Can you work these out from the model? Positions are in its coordinate system, mm. A direction names the side the tool comes from. Round coordinates to 2 decimals unless told otherwise and drop trailing zeros. Write each loop counter-clockwise with the first axis right and the second up, starting at its lowest first coordinate (ties: lowest second). Pieces come first, ordered by that corner, then holes. Notation, with made-up numbers: M 44,81.5 L 79,81.5 A19 cw 79,87.5 Z; hole C 17.5,-23.5 d2. An arc over 180 degrees is marked long. Answer in a Markdown table with one row per item. Add a question column.
(1) For faces 5 (the face through (21.15, 0, -18)), 6 (the face through (-2.38, 10.74, 1.01)), which set-ups out of +Z, -Z, +X, -X, +Y, -Y let a thin tool reach every point of the face, with its end or its side?
(2) Suppose I cut it at D-D, the plane x = -7.5. Write out the boundary of the cut face in (y, z).
(3) Suppose I cut it at A-A, the plane x = 0. Write out the boundary of the cut face in (y, z), then the cut area to 3 significant figures.
(4) If I drill on probe 1 along X at (y, z) = (-15.5, -24.5); probe 2 along Y at (x, z) = (-15, -17), over which ranges is the centre line in solid material (lowest first)?
(5) I'm going to push a flat-ended pin straight in: pin 1 (3 mm diameter, centred on x = 15.5, y = 15.5, fed in from +Z). Where does the tip first touch, or does it pass through?
(6) If we mould it in two halves opening along X, with no side actions, what happens to faces 1 (the face through (0, 0, 24)), 2 (the face through (14.579, -16.345, -18.487)), 3 (the face through (18.42, -18.35, -18.49)), 4 (the face through (-0.54, 2.44, 13.15))? For each: released by +X, released by -X, zero draft, split by the parting line, or undercut.
(7) Suppose I cut it at C-C, the plane z = 1. Write out the boundary of the cut face in (x, y), then the cut area to 3 significant figures.
from build123d import *

# Parameters (mm, degrees)
BOX002_W                    = 100
BOX002_H                    = 100
BOX002_DEPTH                = 37.5
COMPOUND002_PLACEMENT_ANGLE = 135
BOX003_W                    = 100
BOX003_H                    = 100
BOX003_DEPTH                = 37.5
COMPOUND003_PLACEMENT_ANGLE = 225
BOX004_W                    = 100
BOX004_H                    = 100
BOX004_DEPTH                = 37.5
COMPOUND004_PLACEMENT_ANGLE = 315
BOX001_W                    = 100
BOX001_H                    = 100
BOX001_DEPTH                = 37.5
COMPOUND001_PLACEMENT_ANGLE = 45
CYLINDER002_R               = 1.25
CYLINDER002_DEPTH           = 37.5
CYLINDER003_R               = 1.25
CYLINDER003_DEPTH           = 37.5
CYLINDER004_R               = 1.25
CYLINDER004_DEPTH           = 37.5
CYLINDER005_R               = 1.25
CYLINDER005_DEPTH           = 37.5
BOX_W                       = 42.3
BOX_H                       = 42.3
BOX_DEPTH                   = 37.5
CYLINDER_R                  = 11
CYLINDER_DEPTH              = 2
CYLINDER001_R               = 2.5
CYLINDER001_DEPTH           = 24
CUT001_PLACEMENT_ANGLE      = 180


with BuildPart() as compound002:
    # Box002 → Box002 (new body)
    with BuildSketch(Plane(origin=(26, -50, 0), x_dir=(1, 0, 0), z_dir=(0, 0, 1))):
        with Locations((50, 50)):
            Rectangle(BOX002_W, BOX002_H)
    extrude(amount=BOX002_DEPTH)


with BuildPart() as compound002_1:
    # Compound002 placement: moved
    add(compound002.part.rotate(Axis((0, 0, 0), (0, 0, 1)), COMPOUND002_PLACEMENT_ANGLE))


with BuildPart() as compound003:
    # Box003 → Box003 (new body)
    with BuildSketch(Plane(origin=(26, -50, 0), x_dir=(1, 0, 0), z_dir=(0, 0, 1))):
        with Locations((50, 50)):
            Rectangle(BOX003_W, BOX003_H)
    extrude(amount=BOX003_DEPTH)


with BuildPart() as compound003_1:
    # Compound003 placement: moved
    add(compound003.part.rotate(Axis((0, 0, 0), (0, 0, 1)), COMPOUND003_PLACEMENT_ANGLE))


with BuildPart() as compound004:
    # Box004 → Box004 (new body)
    with BuildSketch(Plane(origin=(26, -50, 0), x_dir=(1, 0, 0), z_dir=(0, 0, 1))):
        with Locations((50, 50)):
            Rectangle(BOX004_W, BOX004_H)
    extrude(amount=BOX004_DEPTH)


with BuildPart() as compound004_1:
    # Compound004 placement: moved
    add(compound004.part.rotate(Axis((0, 0, 0), (0, 0, 1)), COMPOUND004_PLACEMENT_ANGLE))


with BuildPart() as compound005:
    # Box001 → Box001 (new body)
    with BuildSketch(Plane(origin=(26, -50, 0), x_dir=(1, 0, 0), z_dir=(0, 0, 1))):
        with Locations((50, 50)):
            Rectangle(BOX001_W, BOX001_H)
    extrude(amount=BOX001_DEPTH)


with BuildPart() as compound005_1:
    # Compound001 placement: moved
    add(compound005.part.rotate(Axis((0, 0, 0), (0, 0, 1)), COMPOUND001_PLACEMENT_ANGLE))

    # Compound005: union Compound002, Compound003, Compound004
    add(compound002_1.part)
    add(compound003_1.part)
    add(compound004_1.part)


with BuildPart() as cylinder002:
    # Cylinder002 → Cylinder002 (new body)
    with BuildSketch(Plane(origin=(15.5, 15.5, 0), x_dir=(1, 0, 0), z_dir=(0, 0, 1))):
        Circle(CYLINDER002_R)
    extrude(amount=CYLINDER002_DEPTH)


with BuildPart() as cylinder003:
    # Cylinder003 → Cylinder003 (new body)
    with BuildSketch(Plane(origin=(-15.5, 15.5, 0), x_dir=(1, 0, 0), z_dir=(0, 0, 1))):
        Circle(CYLINDER003_R)
    extrude(amount=CYLINDER003_DEPTH)


with BuildPart() as cylinder004:
    # Cylinder004 → Cylinder004 (new body)
    with BuildSketch(Plane(origin=(15.5, -15.5, 0), x_dir=(1, 0, 0), z_dir=(0, 0, 1))):
        Circle(CYLINDER004_R)
    extrude(amount=CYLINDER004_DEPTH)


with BuildPart() as compound:
    # Cylinder005 → Cylinder005 (new body)
    with BuildSketch(Plane(origin=(-15.5, -15.5, 0), x_dir=(1, 0, 0), z_dir=(0, 0, 1))):
        Circle(CYLINDER005_R)
    extrude(amount=CYLINDER005_DEPTH)

    # Compound: union Cylinder002, Cylinder003, Cylinder004
    add(cylinder002.part)
    add(cylinder003.part)
    add(cylinder004.part)


with BuildPart() as cube:
    # Box → Box (new body)
    with BuildSketch(Plane(origin=(-21.15, -21.15, 0), x_dir=(1, 0, 0), z_dir=(0, 0, 1))):
        with Locations((21.15, 21.15)):
            Rectangle(BOX_W, BOX_H)
    extrude(amount=BOX_DEPTH)


with BuildPart() as fusion:
    # Cylinder → Cylinder (new body)
    with BuildSketch(Plane.XY.offset(-2)):
        Circle(CYLINDER_R)
    extrude(amount=CYLINDER_DEPTH)

    # Fusion: union Cube
    add(cube.part)


with BuildPart() as nema17stepper:
    # Cylinder001 → Cylinder001 (new body)
    with BuildSketch(Plane.XY.offset(-24)):
        Circle(CYLINDER001_R)
    extrude(amount=CYLINDER001_DEPTH)

    # Fusion001: union Fusion
    add(fusion.part)

    # Cut: cut Compound
    add(compound.part, mode=Mode.SUBTRACT)

    # Cut001: cut Compound005
    add(compound005_1.part, mode=Mode.SUBTRACT)


with BuildPart() as nema17stepper_1:
    # Cut001 placement: moved
    add(nema17stepper.part.rotate(Axis((0, 0, 0), (1, 0, 0)), CUT001_PLACEMENT_ANGLE))


solid = nema17stepper_1.part
Calculated:
| question | item | result |
|---|---|---|
| 1 | face 5 | +Z, -Z, +X, +Y, -Y |
| 1 | face 6 | +Z |
| 2 | outline | M -21.15,-37.5 L 21.15,-37.5 L 21.15,0 L 8.05,0 L 8.05,2 L -8.05,2 L -8.05,0 L -21.15,0 Z |
| 3 | outline | M -21.15,-37.5 L 21.15,-37.5 L 21.15,0 L 11,0 L 11,2 L 2.5,2 L 2.5,24 L -2.5,24 L -2.5,2 L -11,2 L -11,0 L -21.15,0 Z |
| 3 | area | 1,740 mm² |
| 4 | probe 1 | -21.15 to -16.75, -14.25 to 14.25, 16.75 to 21.15 |
| 4 | probe 2 | -21.15 to -16.65, -14.35 to 14.35, 16.65 to 21.15 |
| 5 | pin 1 | z = 0 |
| 6 | face 1 | zero draft |
| 6 | face 2 | undercut |
| 6 | face 3 | released by +X |
| 6 | face 4 | split by the parting line |
| 7 | outline | C 0,0 d22 |
| 7 | area | 380 mm² |
